```python
from build123d import *

# Parameters (mm, degrees)
SKETCH1_W           = 6.35
SKETCH1_H           = 6.35
BOSS_EXTRUDE1_DEPTH = 74.3375
CUT_EXTRUDE1_START  = -4.0132
SKETCH2_W           = 6.604
SKETCH2_H           = 6.604
SKETCH2_R           = 3.175
CUT_EXTRUDE1_DEPTH  = 4.0132


with BuildPart() as part:
    # Sketch1 → Boss-Extrude1 (new body)
    with BuildSketch(Plane(origin=(0, 0, 0), x_dir=(0, 0, -1), z_dir=(1, 0, 0))):
        Rectangle(SKETCH1_W, SKETCH1_H)
    extrude(amount=BOSS_EXTRUDE1_DEPTH)

    # Sketch2 → Cut-Extrude1 (cut)
    with BuildSketch(Plane(origin=(74.3375, 0, 0), x_dir=(0, 0, -1), z_dir=(1, 0, 0)).offset(CUT_EXTRUDE1_START)):
        Rectangle(SKETCH2_W, SKETCH2_H)
        Circle(SKETCH2_R, mode=Mode.SUBTRACT)
    extrude(amount=CUT_EXTRUDE1_DEPTH, mode=Mode.SUBTRACT)


solid = part.part
```
The listing builds one solid part. Answer for the finished solid, in the listing's coordinates (mm). A direction names the side the tool comes from. Coordinates: 2 decimals unless noted, no trailing zeros. Order: outer loops, then holes, each group sorted by start corner. A loop starts at its lowest first (then second) coordinate and runs counter-clockwise, first axis right, second up. Notation, with made-up numbers: M -5.5,-31.5 L 52.5,-31.5 A19 ccw 52.5,-22.5 Z; hole C 36.5,32.25 d5. An arc over 180 degrees is marked long. Answer as a JSON object with one key per item and string values. Group by question number.
1. A tool of negligible diameter and unlimited length cuts with its end or side. For faces 1 (the cylindrical face through (72.3, -3.1, 0.69)), 2 (the flat face through (70.324, -2, 3)), 3 (the flat face through (70.324, -3, -3)), 4 (the flat face through (70.324, 2, 3)), 5 (the flat face through (70.324, 3, -2)), from which of +Z, -Z, +X, -X, +Y, -Y can it reach the whole face along a straight path? Write none if from no direction.
2. Straight lines are drawn through the part: line 1 (X direction, y = -2.5, z = 2.5); line 2 (Y direction, x = 71, z = 1.25). For each, find the intervals that lie inside material, in ascending order.
3. Section A-A on y = -2.5 is taken. Write down the section's boundary in (x, z) (1 decimal), then the cut area to 3 significant figures.
Values follow:
{
 "1": {"face 1": "+X", "face 2": "+Z, +X, -Y", "face 3": "-Z, +X, -Y", "face 4": "+Z, +X, +Y", "face 5": "-Z, +X, +Y"},
 "2": {"line 1": "0 to 70.32", "line 2": "-2.92 to 2.92"},
 "3": {"outline": "M 0,-3.2 L 70.3,-3.2 L 70.3,-2 L 74.3,-2 L 74.3,2 L 70.3,2 L 70.3,3.2 L 0,3.2 Z", "area": "462 mm2"}
}
